Part model, mm, in its own coordinate system. Give positions to 0.01 mm unless a question says otherwise; leave off trailing zeros. Write each loop counter-clockwise with the first axis right and the second up, starting at its lowest first coordinate (ties: lowest second). Pieces come first, ordered by that corner, then holes. Notation, with made-up numbers: M 7.25,-24.75 L 58.25,-24.75 A31 cw 58.25,0.25 Z; hole C -9,-35.75 d7. An arc over 180 degrees is marked long. Answer as CSV lines item,"result". Start each with the question number.
Item 1: Band-saw the part on D-D, the plane x = -60.25. List the corners of the cut face in (y, z).
Item 2: Wall check: L1, parallel to Y at x = -59, z = 7.25; L2, parallel to X at y = 107.75, z = 8; L3, parallel to X at y = 106.25, z = 17.25. Give the ranges that are in metal, low to high. Write a range as from..to.
Item 3: Band-saw the part on A-A, the plane z = 3. List the corners of the cut face in (x, y), then the cut area to 3 significant figures.
Item 4: Band-saw the part on C-C, the plane x = -59. List the corners of the cut face in (y, z) (3 decimals), then the cut area to 3 significant figures.
Item 5: Band-saw the part on B-B, the plane y = 107. List the corners of the cut face in (x, z) (3 decimals).
Item 6: Two-plate mould, pull along X, no slides. Class faces 1 (the flat face through (-58.74, 109.99, 12.32)), 2 (the flat face through (-61.72, 105.73, 12.32)), 3 (the flat face through (-60, 108, 25)), 4 (the cylindrical face through (-58.2, 106.4, 12.3)): +X half, -X half, draft (parallel to the pull), parting line (faces both ways), or undercut.
Item 7: Pin check, flat tips, straight feed: pin 1 (1.2 mm diameter, centred on x = -59, y = 107, fed in from +Z); pin 2 (1 mm diameter, centred on x = -61.5, z = 19.5, fed in from -Y). Stop position of each tip, or through.
from build123d import *

# Parameters (mm, degrees)
BOSS_EXTRUDE1_DEPTH             = 25
F_2_0MM_DOWEL_HOLE1_D           = 2
F_2_0MM_DOWEL_HOLE1_DEPTH       = 25
F_2_0MM_DOWEL_HOLE1_CSINK_D     = 2.05
F_2_0MM_DOWEL_HOLE1_CSINK_ANGLE = 90
F_2_0MM_DOWEL_HOLE1_TIP         = 0.600860619


with BuildPart() as part:
    # Sketch1 → Boss-Extrude1 (new body)
    with BuildSketch(Plane.XY):
        Polygon((-60.488817819, 110.127846144), (-62.453203129, 107.27456902), (-60.964385311, 104.146722875), (-57.511182181, 103.872153856), (-55.546796871, 106.72543098), (-57.035614689, 109.853277125), align=None)
    extrude(amount=BOSS_EXTRUDE1_DEPTH)

    # Ø2.0mm Dowel Hole1
    with Locations(Plane(origin=(-59, 107, 25), x_dir=(1, 0, 0), z_dir=(0, 0, 1))):
        with Locations((0, 0)):
            CounterSinkHole(F_2_0MM_DOWEL_HOLE1_D / 2, F_2_0MM_DOWEL_HOLE1_CSINK_D / 2, depth=F_2_0MM_DOWEL_HOLE1_DEPTH, counter_sink_angle=F_2_0MM_DOWEL_HOLE1_CSINK_ANGLE)
            with Locations((0, 0, -(F_2_0MM_DOWEL_HOLE1_DEPTH + F_2_0MM_DOWEL_HOLE1_TIP / 2))):  # 118° drill point
                Cone(0, F_2_0MM_DOWEL_HOLE1_D / 2, F_2_0MM_DOWEL_HOLE1_TIP, mode=Mode.SUBTRACT)


solid = part.part
Output:
1,outline,"M 104.09,0 L 110.11,0 L 110.11,25 L 104.09,25 Z"
2,L1,"103.99..106, 108..110.01"
2,L2,"-62.13..-59.66, -58.34..-56.03"
2,L3,"-61.97..-59.66, -58.34..-55.87"
3,outline,"M -62.45,107.27 L -60.96,104.15 L -57.51,103.87 L -55.55,106.73 L -57.04,109.85 L -60.49,110.13 Z; hole C -59,107 d2"
3,area,"28.0 mm²"
4,outline,"M 103.991,0 L 106,0 L 106,24.975 L 105.975,25 L 103.991,25 Z; M 108,0 L 110.009,0 L 110.009,25 L 108.025,25 L 108,24.975 Z"
4,area,"100 mm²"
5,outline,"M -62.323,0 L -60,0 L -60,24.975 L -60.025,25 L -62.323,25 Z; M -58,0 L -55.677,0 L -55.677,25 L -57.975,25 L -58,24.975 Z"
6,face 1,"+X half"
6,face 2,"-X half"
6,face 3,"draft"
6,face 4,"undercut"
7,pin 1,"through"
7,pin 2,"y = 104.22"
